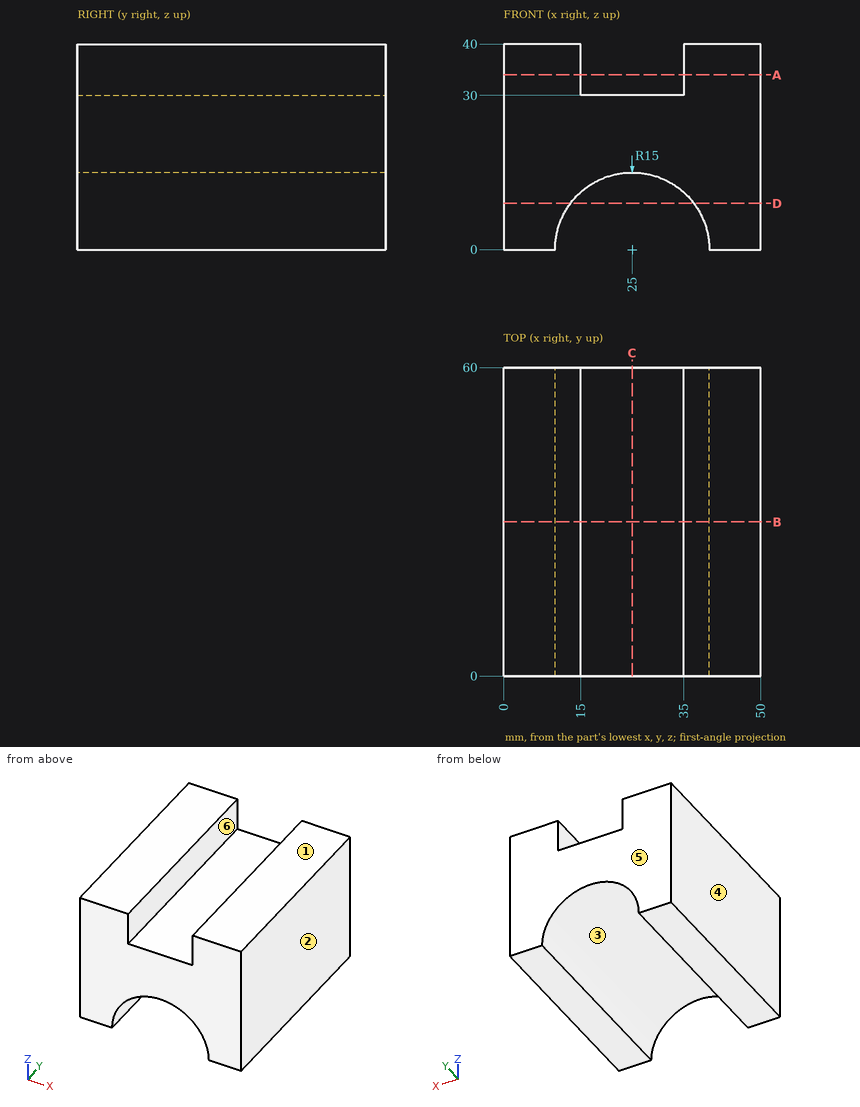
For this review, use the dimensioned drawing (mm, ordinates from the lowest corner) and the shaded views. A direction names the side the tool comes from. Coordinates: 2 decimals unless noted, no trailing zeros. Order: outer loops, then holes, each group sorted by start corner. A loop starts at its lowest first (then second) coordinate and runs counter-clockwise, first axis right, second up. Notation, with made-up numbers: (-25.75, 45) - (-11.75, 45) arc R13 ccw to (-11.75, 57) - close; hole circle Ø7 at (85, 44). An arc over 180 degrees is marked (long way). Answer in a Markdown table with one row per item.
(1) For the marked faces 5 and 6, list the 3-axis set-ups (+Z, -Z, +X, -X, +Y, -Y) from which the entire face can be reached by the end or side of a thin tool; tool diameter is ignored.
Checked values:
| item | result |
|---|---|
| face 5 | +Z, -Z, +X, -X, +Y |
| face 6 | +Z, +Y, -Y |
(2) Clearance check with flat-ended pins moving along their axes: pin 1 (4 mm diameter, centred on x = 26.5, y = 24, fed in from +Z); pin 2 (12 mm diameter, centred on x = 31, y = 21.5, fed in from -Z). State where each tip first meets the part, or that it passes through.
Checked values:
| item | result |
|---|---|
| pin 1 | z = 30 |
| pin 2 | z = 9 |
(3) The part is to be moulded in two halves that separate along X. For the marked faces 1, 2, 3 and 4, say which applies: released by +X, released by -X, zero draft, split by the parting line, or undercut.
Checked values:
| item | result |
|---|---|
| face 1 | zero draft |
| face 2 | released by +X |
| face 3 | undercut |
| face 4 | released by -X |
(4) Consider section C-C on x = 25. State the section outline as (y, z) points.
Checked values:
| item | result |
|---|---|
| outline | (0, 15) - (60, 15) - (60, 30) - (0, 30) - close |
(5) Consider section A-A on z = 34. State the section outline as (x, y) points.
Checked values:
| item | result |
|---|---|
| outline | (0, 0) - (15, 0) - (15, 60) - (0, 60) - close; (35, 0) - (50, 0) - (50, 60) - (35, 60) - close |
(6) Consider section D-D on z = 9. State the section outline as (x, y) points, plus the area to 3 significant figures.
Checked values:
| item | result |
|---|---|
| outline | (0, 0) - (13, 0) - (13, 60) - (0, 60) - close; (37, 0) - (50, 0) - (50, 60) - (37, 60) - close |
| area | 1,560 mm^2 |
(7) Wall thickness on line 1 along X through (y, z) = (7, 38.5); line 2 along X through (y, z) = (56, 4.5); line 3 along Z through (x, y) = (25, 23.5): over which ranges is each line inside the solid? List them lowest first. Write a range as from..to.
Checked values:
| item | result |
|---|---|
| line 1 | 0..15, 35..50 |
| line 2 | 0..10.69, 39.31..50 |
| line 3 | 15..30 |
(8) Consider section B-B on y = 30. State the section outline as (x, z) points.
Checked values:
| item | result |
|---|---|
| outline | (0, 0) - (10, 0) arc R15 cw to (40, 0) - (50, 0) - (50, 40) - (35, 40) - (35, 30) - (15, 30) - (15, 40) - (0, 40) - close |
